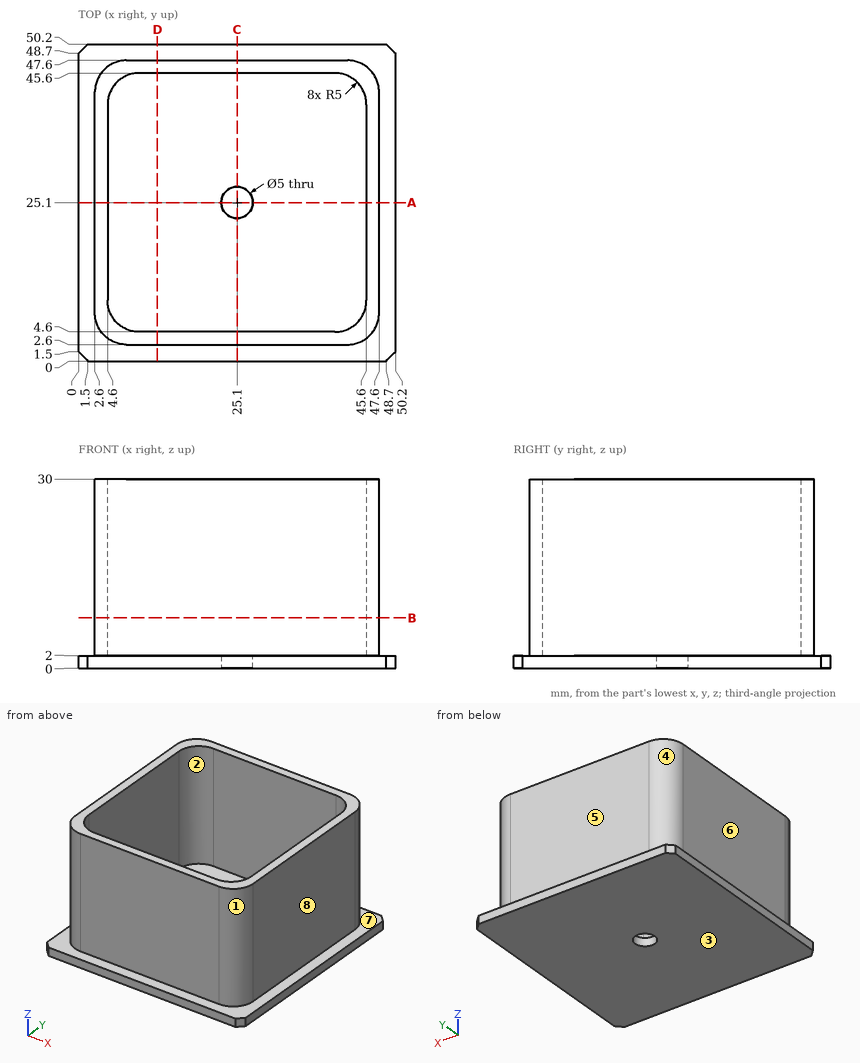
Geometry check sheet. Reference: drawing and pictorial views, mm from the part's lowest x, y, z. A direction names the side the tool comes from. Give positions to 0.01 mm unless a question says otherwise; leave off trailing zeros. Order: outer loops, then holes, each group sorted by start corner. A loop starts at its lowest first (then second) coordinate and runs counter-clockwise, first axis right, second up. Notation, with made-up numbers: M -19.5,45 L 12.5,45 A24 ccw 12.5,71 Z; hole C 87,73.5 d6. An arc over 180 degrees is marked long. Answer as a JSON object with one key per item and string values. Group by question number.
1) Cross-section at B-B (z = 8). Enter the section's corners in (x, y).
2) Depth check by flat-ended pin: pin 1 Ø6 at (y, z) = (36, 23.5) entering from +X; pin 2 Ø14 at (y, z) = (27.5, 9.5) entering from -X; pin 3 Ø5 at (x, z) = (7.5, 12) entering from +Y; pin 4 Ø1 at (x, y) = (7.5, 25.5) entering from -Z. Enter the tip coordinate at first touch or a pass-through.
3) Cross-section at A-A (y = 25.1). Enter the section's corners in (x, z).
4) Cross-section at D-D (x = 12.5). Enter the section's corners in (y, z), then the cut area to 3 significant figures.
5) Scan lines: line 1 along Y through (x, z) = (25.1, 0.7); line 2 along X through (y, z) = (21, 22). Record each from-to range of solid material in increasing order. Write a range as [from, to].
6) Mould release check, pull along Y, two halves, no side actions. Record for the marked faces 1, 2, 3 and 4: released by +Y, released by -Y, zero draft, split by the parting line, or undercut.
7) Access from +Z, -Z, +X, -X, +Y, -Y to the whole of each face (thin tool, end or side, straight path). Record for the marked faces 5, 6, 7 and 8.
Result sheet:
{
 "1": {"outline": "M 2.6,7.6 A5 ccw 7.6,2.6 L 42.6,2.6 A5 ccw 47.6,7.6 L 47.6,42.6 A5 ccw 42.6,47.6 L 7.6,47.6 A5 ccw 2.6,42.6 Z; hole M 4.6,9.6 A5 ccw 9.6,4.6 L 40.6,4.6 A5 ccw 45.6,9.6 L 45.6,40.6 A5 ccw 40.6,45.6 L 9.6,45.6 A5 ccw 4.6,40.6 Z"},
 "2": {"pin 1": "stops at x = 47.6", "pin 2": "stops at x = 2.6", "pin 3": "stops at y = 47.6", "pin 4": "stops at z = 0"},
 "3": {"outline": "M 0,0 L 22.6,0 L 22.6,2 L 4.6,2 L 4.6,30 L 2.6,30 L 2.6,2 L 0,2 Z; M 27.6,0 L 50.2,0 L 50.2,2 L 47.6,2 L 47.6,30 L 45.6,30 L 45.6,2 L 27.6,2 Z"},
 "4": {"outline": "M 0,0 L 50.2,0 L 50.2,2 L 47.6,2 L 47.6,30 L 45.6,30 L 45.6,2 L 4.6,2 L 4.6,30 L 2.6,30 L 2.6,2 L 0,2 Z", "area": "212 mm2"},
 "5": {"line 1": "y = [0, 22.6], [27.6, 50.2]", "line 2": "x = [2.6, 4.6], [45.6, 47.6]"},
 "6": {"face 1": "released by -Y", "face 2": "undercut", "face 3": "zero draft", "face 4": "released by +Y"},
 "7": {"face 5": "+Z, +X, -X, +Y", "face 6": "+Z, -X, +Y, -Y", "face 7": "+Z", "face 8": "+Z, +X, +Y, -Y"}
}
